CAD build for the part. Positions are in the model's coordinates, mm. Face numbers are marked on the shaded views. A direction names the side the tool comes from. Round coordinates to 2 decimals unless told otherwise and drop trailing zeros. Write each loop counter-clockwise with the first axis right and the second up, starting at its lowest first coordinate (ties: lowest second). Pieces come first, ordered by that corner, then holes. Notation, with made-up numbers: (-23, -17.5) - (18, -17.5) arc R32 ccw to (18, 11.5) - close; hole circle Ø9 at (-12.5, -29). An arc over 180 degrees is marked (long way). Use one line per item in the form item = value. Start each with the question number.
Item 1: Pull direction Y, two halves, no side cores. Call the marked faces 3, 4, 5 and 6: +Y half, -Y half, draft (parallel to the pull), parting line (faces both ways), or undercut.
Item 2: Tool access for the marked faces 1 and 2: list every direction of +Z, -Z, +X, -X, +Y, -Y with a clear straight run to the whole face (end or side of a thin tool).
Item 3: Band-saw the part on D-D, the plane z = 13. List the corners of the cut face in (x, y), and give its area (3 significant figures).
Item 4: Drill centre lines: L1, parallel to Z at x = 0, y = 2.2 (3 decimals); L2, parallel to X at y = 2.55, z = 3.75 (3 decimals); L3, parallel to X at y = 0, z = 7 (3 decimals). Where is each one in solid material? Low to high.
Item 5: Band-saw the part on B-B, the plane z = 1.5. List the corners of the cut face in (x, y) (3 decimals), and give its area (3 significant figures).
Item 6: Pin check, flat tips, straight feed: pin 1 (1.5 mm diameter, centred on y = 5.5, z = 5.5, fed in from +X); pin 2 (1.9 mm diameter, centred on x = 0, z = 3.75, fed in from -Y); pin 3 (1.9 mm diameter, centred on x = 0, z = 3.75, fed in from +Y). Stop position of each tip, or through.
Item 7: Band-saw the part on A-A, the plane y = 1. List the corners of the cut face in (x, z) (3 decimals).
Item 8: Band-saw the part on C-C, the plane x = -3.5. List the corners of the cut face in (y, z).
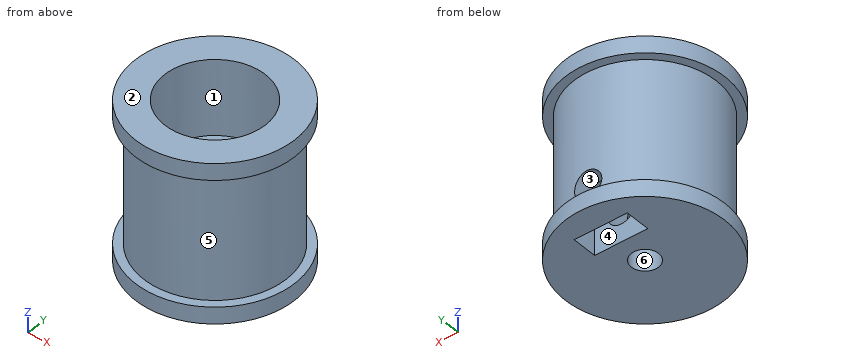
from build123d import *

# Parameters (mm, degrees)
CROQUIS1_R                 = 8.5
SALIENTE_EXTRUIR1_DEPTH    = 19
CROQUIS2_R                 = 1.625
CORTAR_EXTRUIR1_DEPTH      = 1
CORTAR_EXTRUIR1_DEPTH_BACK = 20
CROQUIS3_W                 = 6.34
CROQUIS3_H                 = 3
CORTAR_EXTRUIR2_DEPTH      = 7.5
CROQUIS4_R                 = 9.5
CROQUIS4_R_2               = 8.5
SALIENTE_EXTRUIR2_DEPTH    = 2
CROQUIS5_R                 = 9.5
CROQUIS5_R_2               = 8.5
SALIENTE_EXTRUIR3_DEPTH    = 2
CROQUIS7_R                 = 1.625
CORTAR_EXTRUIR4_DEPTH      = 6.7
CORTAR_EXTRUIR4_DEPTH_BACK = 3
CROQUIS9_R                 = 6
CORTAR_EXTRUIR5_DEPTH      = 9


with BuildPart() as part:
    # Croquis1 → Saliente-Extruir1 (new body)
    with BuildSketch(Plane.XY):
        Circle(CROQUIS1_R)
    extrude(amount=SALIENTE_EXTRUIR1_DEPTH)

    # Croquis2 → Cortar-Extruir1 (cut, two sides)
    with BuildSketch(Plane(origin=(0, 0, 0), x_dir=(-1, 0, 0), z_dir=(0, 0, -1))) as cortar_extruir1_sk:
        Circle(CROQUIS2_R)
    extrude(amount=CORTAR_EXTRUIR1_DEPTH, mode=Mode.SUBTRACT)
    extrude(cortar_extruir1_sk.sketch, amount=-CORTAR_EXTRUIR1_DEPTH_BACK, mode=Mode.SUBTRACT)

    # Croquis3 → Cortar-Extruir2 (cut)
    with BuildSketch(Plane(origin=(0, 0, 0), x_dir=(-1, 0, 0), z_dir=(0, 0, -1))):
        with Locations((0, 5)):
            Rectangle(CROQUIS3_W, CROQUIS3_H)
    extrude(amount=-CORTAR_EXTRUIR2_DEPTH, mode=Mode.SUBTRACT)

    # Croquis4 → Saliente-Extruir2 (add)
    with BuildSketch(Plane(origin=(0, 0, 0), x_dir=(-1, 0, 0), z_dir=(0, 0, -1))):
        Circle(CROQUIS4_R)
        Circle(CROQUIS4_R_2, mode=Mode.SUBTRACT)
    extrude(amount=-SALIENTE_EXTRUIR2_DEPTH)

    # Croquis5 → Saliente-Extruir3 (add)
    with BuildSketch(Plane.XY.offset(19)):
        Circle(CROQUIS5_R)
        Circle(CROQUIS5_R_2, mode=Mode.SUBTRACT)
    extrude(amount=-SALIENTE_EXTRUIR3_DEPTH)

    # Croquis7 → Cortar-Extruir4 (cut, two sides)
    with BuildSketch(Plane.XZ.offset(-6.5)) as cortar_extruir4_sk:
        with Locations((0, 3.75)):
            Circle(CROQUIS7_R)
    extrude(amount=CORTAR_EXTRUIR4_DEPTH, mode=Mode.SUBTRACT)
    extrude(cortar_extruir4_sk.sketch, amount=-CORTAR_EXTRUIR4_DEPTH_BACK, mode=Mode.SUBTRACT)

    # Croquis9 → Cortar-Extruir5 (cut)
    with BuildSketch(Plane.XY.offset(19)):
        Circle(CROQUIS9_R)
    extrude(amount=-CORTAR_EXTRUIR5_DEPTH, mode=Mode.SUBTRACT)


solid = part.part
Determined:
q1.face_3 = draft
q1.face_4 = undercut
q1.face_5 = parting line
q1.face_6 = undercut
q2.face_1 = +Z
q2.face_2 = +Z, +X, -X, +Y, -Y
q3.outline = circle Ø17 at (0, 0); hole circle Ø12 at (0, 0)
q3.area = 114 mm²
q4.L1 = 0 to 2.125, 5.375 to 10
q4.L2 = -8.108 to -1.625, 1.625 to 8.108
q4.L3 = -8.5 to -1.625, 1.625 to 8.5
q5.outline = circle Ø19 at (0, 0); hole (-3.17, 3.5) - (3.17, 3.5) - (3.17, 6.5) - (-3.17, 6.5) - close; hole circle Ø3.25 at (0, 0)
q5.area = 256 mm²
q6.pin_1 = 7.05
q6.pin_2 = -8.5
q6.pin_3 = -1.32
q7.outline = (-9.447, 0) - (-1.281, 0) - (-1.281, 2.75) arc R1.625 cw to (-1.281, 4.75) - (-1.281, 10) - (-5.916, 10) - (-5.916, 19) - (-9.447, 19) - (-9.447, 17) - (-8.441, 17) - (-8.441, 2) - (-9.447, 2) - close; (1.281, 0) - (9.447, 0) - (9.447, 2) - (8.441, 2) - (8.441, 17) - (9.447, 17) - (9.447, 19) - (5.916, 19) - (5.916, 10) - (1.281, 10) - (1.281, 4.75) arc R1.625 cw to (1.281, 2.75) - close
q8.outline = (-8.83, 0) - (8.83, 0) - (8.83, 2) - (7.75, 2) - (7.75, 17) - (8.83, 17) - (8.83, 19) - (4.87, 19) - (4.87, 10) - (-4.87, 10) - (-4.87, 19) - (-8.83, 19) - (-8.83, 17) - (-7.75, 17) - (-7.75, 2) - (-8.83, 2) - close
